Work out the finished part from the listing and answer in its coordinate system (mm). A direction names the side the tool comes from. Round coordinates to 2 decimals unless told otherwise and drop trailing zeros. Write each loop counter-clockwise with the first axis right and the second up, starting at its lowest first coordinate (ties: lowest second). Pieces come first, ordered by that corner, then holes. Notation, with made-up numbers: (-13.5, 80) - (0.5, 80) arc R29 cw to (0.5, 111) - close; hole circle Ø5 at (65, 48). An arc over 180 degrees is marked (long way). Answer as a JSON object with one key per item and string values.
```python
from build123d import *

# Parameters (mm, degrees)
EXTRUDE_1_DEPTH = 2
EXTRUDE_2_DEPTH = 4


with BuildPart() as part:
    # 草图1 → 凸台-拉伸1 (new body)
    with BuildSketch(Plane(origin=(0, 0, 0), x_dir=(1, 0, 0), z_dir=(0, 1, 0))):
        with BuildLine():
            Line((-10.36417176, 0.953563282), (-0.75738839, 0.953563282))
            ThreePointArc((-0.75738839, 0.953563282), (4.168182633, -3.972007741), (-0.75738839, -8.897578764))
            Line((-0.75738839, -8.897578764), (-10.36417176, -8.897578764))
            ThreePointArc((-10.36417176, -8.897578764), (-15.289742784, -3.972007741), (-10.36417176, 0.953563282))
        make_face()
    extrude(amount=EXTRUDE_1_DEPTH)

    # 草图2 → 凸台-拉伸2 (add)
    with BuildSketch(Plane(origin=(0, 2, 0), x_dir=(1, 0, 0), z_dir=(0, 1, 0))):
        with BuildLine():
            Line((-8.92046187, -0.998228401), (-1.597644475, -0.998228401))
            ThreePointArc((-1.597644475, -0.998228401), (1.331482483, -3.927355359), (-1.597644475, -6.856482317))
            Line((-1.597644475, -6.856482317), (-8.92046187, -6.856482317))
            ThreePointArc((-8.92046187, -6.856482317), (-11.849588828, -3.927355359), (-8.92046187, -0.998228401))
        make_face()
    extrude(amount=EXTRUDE_2_DEPTH)


solid = part.part
```
Item 1: Each of these flat-tipped pins is pushed along its axis until it touches: P1, Ø1, axis at y = 0.5, z = 7, coming from the +X side; P2, Ø2, axis at x = -13, y = 1.5, coming from the -Z side; P3, Ø3, axis at x = -5, y = 4.5, coming from the +Z side. Where does it stop, or does it pass through?
Results found:
{"P1": "x = 3.47", "P2": "z = -0.67", "P3": "z = 6.86"}
Item 2: A cutting plane is placed at C-C (y = 3.4). Write down the section's boundary in (x, z), and give its area (3 significant figures).
Results found:
{"outline": "(-8.92, 1) - (-1.6, 1) arc R2.93 ccw to (-1.6, 6.86) - (-8.92, 6.86) arc R2.93 ccw to start", "area": "69.9 mm²"}
Item 3: A cutting plane is placed at B-B (z = 1.25). Write down the section's boundary in (x, y), and give its area (3 significant figures).
Results found:
{"outline": "(-14.47, 0) - (3.35, 0) - (3.35, 2) - (-0.41, 2) - (-0.41, 6) - (-10.11, 6) - (-10.11, 2) - (-14.47, 2) - close", "area": "74.4 mm²"}
Item 4: For faces 1 (the flat face through (-5.4, 2, 7.2)), 2 (the flat face through (-5, 4, 0.998)), 3 (the cylindrical face through (1.33, 3.97, 3.86)), determine the directions among +Z, -Z, +X, -X, +Y, -Y from which every point of the face is accessible in a straight line to the end or side of a thin tool.
Results found:
{"face 1": "+Y", "face 2": "-Z, +X, -X, +Y", "face 3": "+X, +Y"}
Item 5: Consider line 1 along Y through (x, z) = (-13, 4.75); line 2 along Z through (x, y) = (-7.5, 2.55); line 3 along X through (y, z) = (4.2, 2.5). Determine where each line is inside the solid, lowest interval first.
Results found:
{"line 1": "0 to 2", "line 2": "1 to 6.86", "line 3": "-11.48 to 0.96"}
Item 6: A cutting plane is placed at A-A (x = -11.5). Write down the section's boundary in (y, z), and give its area (3 significant figures).
Results found:
{"outline": "(0, -0.82) - (2, -0.82) - (2, 2.54) - (6, 2.54) - (6, 5.32) - (2, 5.32) - (2, 8.76) - (0, 8.76) - close", "area": "30.3 mm²"}
